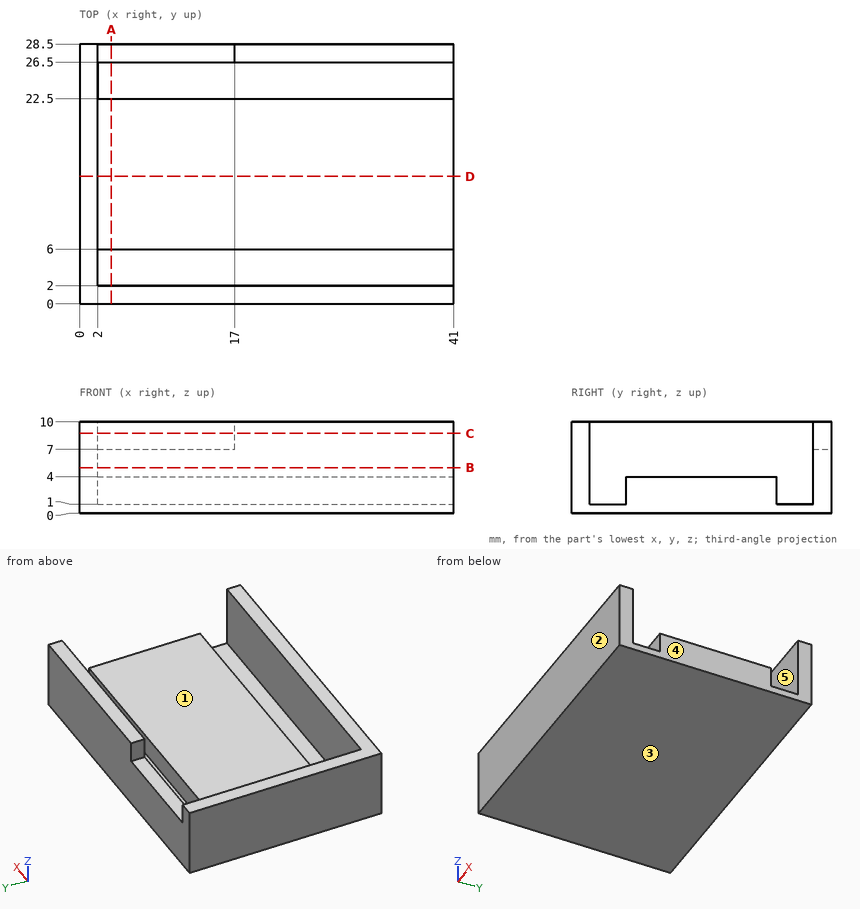
Drawing for the job (mm, zero at the part's lowest x, y, z). A direction names the side the tool comes from. Give positions to 0.01 mm unless a question says otherwise; leave off trailing zeros. Loops run counter-clockwise (first coordinate to the right, second up) from the corner with the lowest first, then second, coordinate; pieces in that order, holes last.
1) Two-plate mould, pull along Y, no slides. Class the marked faces 1, 2 and 3: released by +Y, released by -Y, zero draft, split by the parting line, or undercut.
Values follow:
face 1: undercut
face 2: released by -Y
face 3: zero draft
2) Band-saw the part on B-B on z = 5. List the corners of the cut face in (x, y).
Values follow:
outline: (0, 0) - (41, 0) - (41, 2) - (2, 2) - (2, 26.5) - (41, 26.5) - (41, 28.5) - (0, 28.5) - close
3) Band-saw the part on D-D on y = 14. List the corners of the cut face in (x, z), then the cut area to 3 significant figures.
Values follow:
outline: (0, 0) - (41, 0) - (41, 4) - (2, 4) - (2, 10) - (0, 10) - close
area: 176 mm2
4) Band-saw the part on A-A on x = 3.5. List the corners of the cut face in (y, z), then the cut area to 3 significant figures.
Values follow:
outline: (0, 0) - (28.5, 0) - (28.5, 7) - (26.5, 7) - (26.5, 1) - (22.5, 1) - (22.5, 4) - (6, 4) - (6, 1) - (2, 1) - (2, 10) - (0, 10) - close
area: 108 mm2
5) 3-axis set-ups, long thin cutter, end or side, ignore diameter. For the marked faces 4 and 5: which of +Z, -Z, +X, -X, +Y, -Y reach the whole face in a straight line?
Values follow:
face 4: +Z, -Z, +X, +Y, -Y
face 5: +Z, +X
6) Drop flat-ended pins along their axis: P1, Ø2.5, axis at y = 10.5, z = 6, coming from the +X side; P2, Ø1.2, axis at x = 22.5, y = 4, coming from the +Z side; P3, Ø8, axis at x = 14, y = 14.5, coming from the +Z side. Give the stop position or say it passes through.
Values follow:
P1: stops at x = 2
P2: stops at z = 1
P3: stops at z = 4
7) Band-saw the part on C-C on z = 8.75. List the corners of the cut face in (x, y), then the cut area to 3 significant figures.
Values follow:
outline: (0, 0) - (41, 0) - (41, 2) - (2, 2) - (2, 28.5) - (0, 28.5) - close; (17, 26.5) - (41, 26.5) - (41, 28.5) - (17, 28.5) - close
area: 183 mm2
8) Probe line 1 along Y through (x, z) = (39, 2.75); line 2 along Y through (x, z) = (4, 5.25); line 3 along X through (y, z) = (10.25, 5.75). List the from-to ranges inside material, lowest first.
Values follow:
line 1: y = 0 to 2, 6 to 22.5, 26.5 to 28.5
line 2: y = 0 to 2, 26.5 to 28.5
line 3: x = 0 to 2
